Source: CAD feature listing. Evaluate the final solid. Frame: model axes, mm. Face numbers are marked on the shaded views. Coordinates: 2 decimals unless noted, no trailing zeros. Order: outer loops, then holes, each group sorted by start corner. A loop starts at its lowest first (then second) coordinate and runs counter-clockwise, first axis right, second up. Notation, with made-up numbers: (1.5, 20.25) -> (7.5, 20.25) arc R14 ccw to (7.5, 39.25) -> close; hole circle Ø9 at (-14.75, 58.25). An arc over 180 degrees is marked (long way). Write item = value, one per line. Start each with the question number.
Item 1: Section query C-C (z = 4.75). Output: boundary loops of the cut face in (x, y).
Item 2: Mould query, pull axis Z, two halves, no side actions, for the marked faces 1, 2 and 3. Classes: released by +Z, released by -Z, zero draft, split by the parting line, or undercut.
Item 3: Ray query, line 1 along X through (y, z) = (3.2, 0); line 2 along X through (y, z) = (3.6, 0.75); line 3 along Z through (x, y) = (7, 2). Return the intervals inside material, ascending. Write a range as [from, to].
Item 4: Section query A-A (x = -6). Output: boundary loops of the cut face in (y, z), then the cut area to 3 significant figures.
Item 5: Section query B-B (z = 0). Output: boundary loops of the cut face in (x, y).
Item 6: Section query D-D (y = 3.8). Output: boundary loops of the cut face in (x, z).
```python
from build123d import *

# Parameters (mm, degrees)
SKETCH1_W           = 20
SKETCH1_H           = 12
SKETCH1_R           = 5.1
SKETCH1_R_2         = 1.1
BOSS_EXTRUDE1_DEPTH = 5
FILLET1_R           = 1


with BuildPart() as part:
    # Sketch1 → Boss-Extrude1 (new body)
    with BuildSketch(Plane(origin=(0, 0, 0), x_dir=(1, 0, 0), z_dir=(0, 1, 0))):
        Rectangle(SKETCH1_W, SKETCH1_H)
        with Locations(Location((-2.32697534, 0, 0), (0, 0, 270))):
            Circle(SKETCH1_R, mode=Mode.SUBTRACT)
        with Locations(Location((7.67302466, 0, 0), (0, 0, 270))):
            Circle(SKETCH1_R_2, mode=Mode.SUBTRACT)
    extrude(amount=BOSS_EXTRUDE1_DEPTH)

    # Fillet1
    fillet1_edges = [part.edges().sort_by_distance(p)[0] for p in [
        (-10, 2.5, -6),
        (10, 2.5, -6),
        (10, 2.5, 6),
        (-10, 2.5, 6),
    ]]
    fillet(fillet1_edges, radius=FILLET1_R)


solid = part.part
```
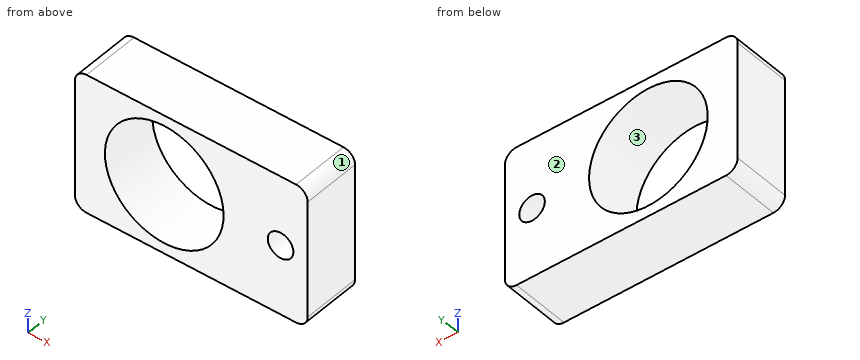
Computed:
q1.outline = (-10, 0) -> (-4.18, 0) -> (-4.18, 5) -> (-10, 5) -> close; (-0.47, 0) -> (10, 0) -> (10, 5) -> (-0.47, 5) -> close
q2.face_1 = released by +Z
q2.face_2 = zero draft
q2.face_3 = undercut
q3.line_1 = [-10, -7.43], [2.77, 6.57], [8.77, 10]
q3.line_2 = [-10, -7.37], [2.72, 6.87], [8.48, 10]
q3.line_3 = [-6, -0.87], [0.87, 6]
q4.outline = (0, -6) -> (5, -6) -> (5, -3.54) -> (0, -3.54) -> close; (0, 3.54) -> (5, 3.54) -> (5, 6) -> (0, 6) -> close
q4.area = 24.6 mm^2
q5.outline = (-10, 0) -> (-7.43, 0) -> (-7.43, 5) -> (-10, 5) -> close; (2.77, 0) -> (6.57, 0) -> (6.57, 5) -> (2.77, 5) -> close; (8.77, 0) -> (10, 0) -> (10, 5) -> (8.77, 5) -> close
q6.outline = (-10, -5) arc R1 ccw to (-9, -6) -> (9, -6) arc R1 ccw to (10, -5) -> (10, 5) arc R1 ccw to (9, 6) -> (-9, 6) arc R1 ccw to (-10, 5) -> close; hole circle Ø10.2 at (-2.33, 0); hole circle Ø2.2 at (7.67, 0)
